from build123d import *

# Parameters (mm, degrees)
SKETCH1_W           = 55.6
SKETCH1_H           = 55.6
BOSS_EXTRUDE1_DEPTH = 23.1
SKETCH2_R           = 25
BOSS_EXTRUDE2_DEPTH = 18.2
SKETCH3_R           = 1.5
CUT_EXTRUDE1_DEPTH  = 7


with BuildPart() as part:
    # Sketch1 → Boss-Extrude1 (new body)
    with BuildSketch(Plane(origin=(0, 0, 0), x_dir=(1, 0, 0), z_dir=(0, 1, 0))):
        Rectangle(SKETCH1_W, SKETCH1_H)
    extrude(amount=BOSS_EXTRUDE1_DEPTH)

    # Sketch2 → Boss-Extrude2 (add)
    with BuildSketch(Plane(origin=(0, 23.1, 0), x_dir=(1, 0, 0), z_dir=(0, 1, 0))):
        with Locations(Location((0, 0, 0), (0, 0, 270))):
            Circle(SKETCH2_R)
    extrude(amount=BOSS_EXTRUDE2_DEPTH)

    # Sketch3 → Cut-Extrude1 (cut)
    with BuildSketch(Plane.XZ):
        with Locations(Location((-21.5, 21.5, 0), (0, 0, 270))):
            Circle(SKETCH3_R)
        with Locations(Location((21.5, 21.5, 0), (0, 0, 270))):
            Circle(SKETCH3_R)
        with Locations(Location((-21.5, -21.5, 0), (0, 0, 270))):
            Circle(SKETCH3_R)
        with Locations(Location((21.5, -21.5, 0), (0, 0, 270))):
            Circle(SKETCH3_R)
    extrude(amount=-CUT_EXTRUDE1_DEPTH, mode=Mode.SUBTRACT)


solid = part.part
For this review, take the finished solid that the model builds, in its own axes (mm). A direction names the side the tool comes from. Round coordinates to 2 decimals unless told otherwise and drop trailing zeros. Loops run counter-clockwise (first coordinate to the right, second up) from the corner with the lowest first, then second, coordinate; pieces in that order, holes last. Notation, with made-up numbers: (31.25, 75) - (55.25, 75) arc R22 cw to (55.25, 104) - close; hole circle Ø4 at (2.25, 4). An arc over 180 degrees is marked (long way). One line per item, written item: value. Start each with the question number.
Item 1: Clearance check with flat-ended pins moving along their axes: pin 1 Ø1.5 at (x, z) = (12.5, -7) entering from -Y; pin 2 Ø2.5 at (x, z) = (-21.5, -21.5) entering from -Y; pin 3 Ø10 at (x, y) = (11, 28.5) entering from +Z; pin 4 Ø3.5 at (x, z) = (-21.5, 21.5) entering from +Y. State where each tip first meets the part, or that it passes through.
Item 2: The part is to be moulded in two halves that separate along X. For faces 4 (the cylindrical face through (7.509, 32.073, 23.846)), 5 (the flat face through (0, 41.3, 0)), 6 (the cylindrical face through (22.51, 3.45, -20.39)), say which applies: +X half, -X half, draft (parallel to the pull), parting line (faces both ways), or undercut.
Item 3: For L1, parallel to X at y = 5.75, z = 21.5; L2, parallel to X at y = 3, z = 21, list the stretches that pass through material, from the lowest coordinate up.
Item 4: Take a section at A-A (x = 0). Give the boundary of the cut face in (y, z), plus the area to 3 significant figures.
Item 5: Take a section at C-C (y = 31). Give the boundary of the cut face in (x, z), plus the area to 3 significant figures.
Item 6: Take a section at B-B (z = -1). Give the boundary of the cut face in (x, y), plus the area to 3 significant figures.
Item 7: For faces 1 (the flat face through (-27.8, 11, 0)), 2 (the flat face through (-21, 7, 22)), 3 (the flat face through (-25, 23.1, -7)), list the 3-axis set-ups (+Z, -Z, +X, -X, +Y, -Y) from which the entire face can be reached by the end or side of a thin tool; tool diameter is ignored.
Item 8: Take a section at D-D (x = -21.5). Give the boundary of the cut face in (y, z).
Answer below:
1. pin 1: stops at y = 0
1. pin 2: stops at y = 7
1. pin 3: stops at z = 24.27
1. pin 4: stops at y = 23.1
2. face 4: parting line
2. face 5: draft
2. face 6: undercut
3. L1: x = -27.8 to -23, -20 to 20, 23 to 27.8
3. L2: x = -27.8 to -22.91, -20.09 to 20.09, 22.91 to 27.8
4. outline: (0, -27.8) - (23.1, -27.8) - (23.1, -25) - (41.3, -25) - (41.3, 25) - (23.1, 25) - (23.1, 27.8) - (0, 27.8) - close
4. area: 2,190 mm2
5. outline: circle Ø50 at (0, 0)
5. area: 1,960 mm2
6. outline: (-27.8, 0) - (27.8, 0) - (27.8, 23.1) - (24.98, 23.1) - (24.98, 41.3) - (-24.98, 41.3) - (-24.98, 23.1) - (-27.8, 23.1) - close
6. area: 2,190 mm2
7. face 1: +Z, -Z, -X, +Y, -Y
7. face 2: -Y
7. face 3: +Y
8. outline: (0, -27.8) - (23.1, -27.8) - (23.1, -12.76) - (41.3, -12.76) - (41.3, 12.76) - (23.1, 12.76) - (23.1, 27.8) - (0, 27.8) - (0, 23) - (7, 23) - (7, 20) - (0, 20) - (0, -20) - (7, -20) - (7, -23) - (0, -23) - close
